Geometry check sheet. Reference: the model listing, model coordinates, mm. A direction names the side the tool comes from. Round coordinates to 2 decimals unless told otherwise and drop trailing zeros. Write each loop counter-clockwise with the first axis right and the second up, starting at its lowest first coordinate (ties: lowest second). Pieces come first, ordered by that corner, then holes. Notation, with made-up numbers: (30.5, 28) -> (48.5, 28) arc R23 cw to (48.5, 67) -> close; hole circle Ø8 at (70.25, 83.5). An arc over 180 degrees is marked (long way). Use a Markdown table: item, result.
Autodesk Inventor part; units mm, degrees
ref_plane "YZ Plane" through (0, 0, 0) normal (1, 0, 0) x (0, 1, 0)
ref_plane "XZ Plane" through (0, 0, 0) normal (0, 1, 0) x (-1, 0, 0)
ref_plane "XY Plane" through (0, 0, 0) normal (0, 0, 1) x (1, 0, 0)
sketch "Sketch2" plane through (0, 0, 0) normal (0, 0, 1) x (1, 0, 0)
  line L0 (0, 0) -> (0, 30)
  line L1 (0, 30) -> (-50, 30)
  line L2 (-50, 30) -> (-50, 0)
  line L3 (-50, 0) -> (0, 0)
  dimension "d10" = 30
  dimension "d30" = 50
extrude "Plate1" add sketch "Sketch2" along normal blind 2
sketch "Sketch3" plane through (-50, 28, 0) normal (0, 1, 0) x (-1, 0, 0)
  line L0 (-50, 0) -> (0, 0)
  line L1 (0, 0) -> (0, 20)
  line L2 (0, 20) -> (-50, 20)
  line L3 (-50, 20) -> (-50, 0)
edge flange "Flange1" height 20 angle 90 thickness 2 bend radius 2.75 thickness toward (0, 1, 0) relief round relief width 2 relief depth 1 edges at (-25, 30, 2) wall of the first edge with corners at (0, 28, 0) (-50, 28, 0) (-50, 28, 20) (0, 28, 20)
bend "Bend1"
corner "Corner1"
fillet "Corner Round1" radius 6 2 edges at (-50, 0, 1) (-50, 29, 20)
sketch "Sketch4" plane through (0, 0, 0) normal (0, 0, -1) x (-1, 0, 0)
  circle A0 centre (39, 15) radius 5
  line L0 (44, 0) -> (0, 0)
  dimension "d25" = 10
  dimension "d26" = 15
  dimension "d27" = 5
extrude "Cut1" cut sketch "Sketch4" against normal blind 2
equation "\"d28\" = Thickness"
equation "\"d7\" = Thickness"
equation "\"d14\" = BendReliefWidth"
equation "\"d15\" = BendReliefDepth"
equation "\"d16\" = MinimumRemnant"
equation "\"d17\" = TransitionRadius"
equation "\"d20\" = BendRadius"
equation "\"d21\" = CornerReliefSize"
equation "\"d22\" = GapSize"
equation "\"d23\" = JacobiRadiusSize"
equation "\"BendReliefWidth\" = Thickness"
equation "\"BendReliefDepth\" = 0.5 * Thickness"
equation "\"CornerReliefSize\" = 4 * Thickness"
equation "\"MinimumRemnant\" = 2 * Thickness"
equation "\"TransitionRadius\" = BendRadius"
equation "\"JacobiRadiusSize\" = BendRadius"
equation "\"GapSize\" = Thickness"
properties part number "MSC 124 ROСKET PILLAR" material "Stainless Steel"
(1) Thickness scan on line 1 (Z direction, x = -13, y = 23); line 2 (Y direction, x = -18, z = 7.5); line 3 (Y direction, x = -39, z = 1.4). Record the ranges inside material, lowest first.
A:
| item | result |
|---|---|
| line 1 | z = 0 to 2 |
| line 2 | y = 28 to 30 |
| line 3 | y = 0 to 10, 20 to 28.62 |
(2) Section check B-B on x = -39. Record the cut outline in (y, z).
A:
| item | result |
|---|---|
| outline | (0, 0) -> (10, 0) -> (10, 2) -> (0, 2) -> close; (20, 0) -> (25.25, 0) arc R4.75 ccw to (30, 4.75) -> (30, 20) -> (28, 20) -> (28, 4.75) arc R2.75 cw to (25.25, 2) -> (20, 2) -> close |
(3) Access from +Z, -Z, +X, -X, +Y, -Y to the whole of each face (thin tool, end or side, straight path). Record for faces 1 (the face through (-25, 13, 2)), 2 (the face through (-22, 29, 20)).
A:
| item | result |
|---|---|
| face 1 | +Z, +X, -X, -Y |
| face 2 | +Z, +X, -X, +Y, -Y |
(4) Section check C-C on x = -8. Record the cut outline in (y, z).
A:
| item | result |
|---|---|
| outline | (0, 0) -> (25.25, 0) arc R4.75 ccw to (30, 4.75) -> (30, 20) -> (28, 20) -> (28, 4.75) arc R2.75 cw to (25.25, 2) -> (0, 2) -> close |
(5) Section check A-A on y = 11. Record the cut outline in (x, z), plus the area to 3 significant figures.
A:
| item | result |
|---|---|
| outline | (-50, 0) -> (-42, 0) -> (-42, 2) -> (-50, 2) -> close; (-36, 0) -> (0, 0) -> (0, 2) -> (-36, 2) -> close |
| area | 88.0 mm2 |
(6) Gauge pin test, flat ends, axial feed: pin 1 Ø1 at (x, y) = (-5.5, 8) entering from +Z; pin 2 Ø2 at (x, z) = (-29, 8.5) entering from -Y; pin 3 Ø2 at (x, z) = (-21.5, 2.5) entering from +Y. Record the tip position at first contact, or that the pin passes through.
A:
| item | result |
|---|---|
| pin 1 | stops at z = 2 |
| pin 2 | stops at y = 28 |
| pin 3 | stops at y = 29.83 |
(7) Release check for a two-part mould opening along X. For faces 3 (the face through (-22, 0, 1)), 4 (the face through (-48.289, 1.804, 1.014)), 5 (the face through (-35, 12, 1)) record: +X half, -X half, draft (parallel to the pull), parting line (faces both ways), or undercut.
A:
| item | result |
|---|---|
| face 3 | draft |
| face 4 | -X half |
| face 5 | undercut |
(8) Section check D-D on y = 15. Record the cut outline in (x, z).
A:
| item | result |
|---|---|
| outline | (-50, 0) -> (-44, 0) -> (-44, 2) -> (-50, 2) -> close; (-34, 0) -> (0, 0) -> (0, 2) -> (-34, 2) -> close |
